Design review of the part built by this model. Coordinates are the model's own, in mm. Face numbers are marked on the shaded views. A direction names the side the tool comes from. Coordinates: 2 decimals unless noted, no trailing zeros. Loops run counter-clockwise (first coordinate to the right, second up) from the corner with the lowest first, then second, coordinate; pieces in that order, holes last. Notation, with made-up numbers: (46, -38.5) -> (75, -38.5) arc R5 ccw to (75, -34.5) -> close; hole circle Ø2 at (80, 70). An arc over 180 degrees is marked (long way). One line per item, written item: value. Start each with the question number.
1. Add section B-B on y = 15. Write out the cut boundary in (x, z).
2. Add section C-C on z = 3. Write out the cut boundary in (x, y), plus the area to 3 significant figures.
3. Add section A-A on z = -2.5. Write out the cut boundary in (x, y), plus the area to 3 significant figures.
4. Machinability: for the marked faces 1 and 2, which of the approach directions +Z, -Z, +X, -X, +Y, -Y give a long, thin tool a straight path to every point of the face, cutting with its end or side? Answer none if there is none.
5. Insertion check: pin 1 (2.5 mm diameter, centred on y = 11.14, z = 21.82, fed in from -X); pin 2 (1 mm diameter, centred on x = -1.5, y = -0.5, fed in from +Z); pin 3 (2 mm diameter, centred on y = 15, z = 25, fed in from -X); pin 4 (1.5 mm diameter, centred on x = -0.5, z = 19, fed in from +Y). Each pin has a flat end and moves straight along its axis. Give the tip position at first contact, or say it passes through.
6. For probe 1 along Z at (x, y) = (-0.35, 16); probe 2 along Z at (x, y) = (-1.25, 14); probe 3 along Y at (x, z) = (0.65, 18.5), list the stretches that pass through material, from the lowest coordinate up.
7. Add section D-D on x = -1.9. Write out the cut boundary in (y, z) (3 decimals).
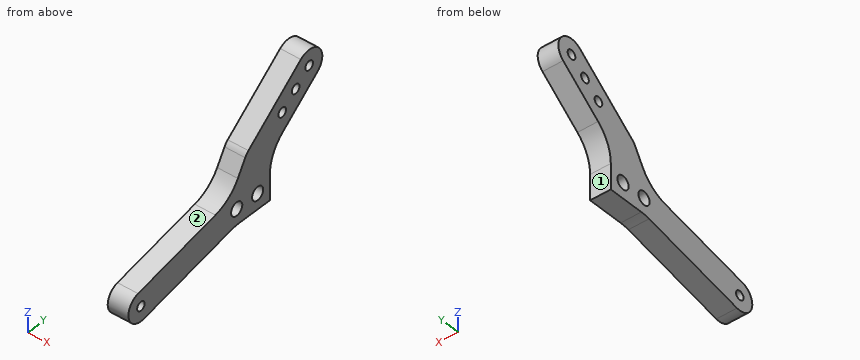
```python
from build123d import *

# Parameters (mm, degrees)
SKETCH1_W           = 5
SKETCH1_H           = 7.5
BOSS_EXTRUDE1_DEPTH = 13
BOSS_EXTRUDE4_DEPTH = 5
SKETCH2_R           = 1.1
CUT_EXTRUDE1_DEPTH  = 35.686092314
LPATTERN1_COUNT     = 3
LPATTERN1_PITCH     = 5
SKETCH3_R           = 1.6
CUT_EXTRUDE2_DEPTH  = 35.686092314
BOSS_EXTRUDE2_DEPTH = 5
LPATTERN2_COUNT     = 2
LPATTERN2_PITCH     = 6
SKETCH5_R           = 1.075
SKETCH5_R_2         = 1.6
BOSS_EXTRUDE3_DEPTH = 5
FILLET2_R           = 10


with BuildPart() as part:
    # Sketch1 → Boss-Extrude1 (new body)
    with BuildSketch(Plane.XY):
        Rectangle(SKETCH1_W, SKETCH1_H)
    extrude(amount=BOSS_EXTRUDE1_DEPTH)

    # Sketch6 → Boss-Extrude4 (add)
    with BuildSketch(Plane(origin=(2.5, 0, 0), x_dir=(0, 0, -1), z_dir=(1, 0, 0))):
        with BuildLine():
            Line((-15.501719728, -2.388104729), (-27.89127235, 12.611895271))
            ThreePointArc((-27.89127235, 12.611895271), (-27.388104729, 17.89127235), (-22.10872765, 17.388104729))
            Line((-22.10872765, 17.388104729), (-9.719175027, 2.388104729))
            ThreePointArc((-9.719175027, 2.388104729), (-10.222342649, -2.89127235), (-15.501719728, -2.388104729))
        make_face()
    extrude(amount=-BOSS_EXTRUDE4_DEPTH)

    # Sketch2 → Cut-Extrude1 (cut, through all)
    with BuildSketch(Plane(origin=(2.5, 0, 0), x_dir=(0, 0, -1), z_dir=(1, 0, 0))):
        with Locations((-25, 15)):
            Circle(SKETCH2_R)
    cut_extrude1 = extrude(amount=-CUT_EXTRUDE1_DEPTH, mode=Mode.SUBTRACT)

    # LPattern1: Cut-Extrude1 ×3
    with Locations(*[Vector(0, -0.7710059601120912, -0.6368279276787667) * (i * LPATTERN1_PITCH) for i in range(1, LPATTERN1_COUNT)]):
        add(cut_extrude1, mode=Mode.SUBTRACT)

    # Sketch3 → Cut-Extrude2 (cut, through all)
    with BuildSketch(Plane(origin=(2.5, 0, 0), x_dir=(0, 0, -1), z_dir=(1, 0, 0))):
        with Locations((-3.75, 0.25)):
            Circle(SKETCH3_R)
    cut_extrude2 = extrude(amount=-CUT_EXTRUDE2_DEPTH, mode=Mode.SUBTRACT)

    # Sketch4 → Boss-Extrude2 (add)
    with BuildSketch(Plane(origin=(2.5, 0, 0), x_dir=(0, 0, -1), z_dir=(1, 0, 0))):
        Polygon((0, -3.75), (0, -8.75), (-5, -8.75), (-14.382714397, -3.304779813), align=None)
    extrude(amount=-BOSS_EXTRUDE2_DEPTH)

    # LPattern2: Cut-Extrude2 ×2
    with Locations(*[(0, -i * LPATTERN2_PITCH, 0) for i in range(1, LPATTERN2_COUNT)]):
        add(cut_extrude2, mode=Mode.SUBTRACT)

    # Sketch5 → Boss-Extrude3 (add)
    with BuildSketch(Plane(origin=(2.5, 0, 0), x_dir=(0, 0, -1), z_dir=(1, 0, 0))):
        with BuildLine():
            Line((-0.985537893, -33.954911928), (-7.235537893, -6.544764489))
            ThreePointArc((-7.235537893, -6.544764489), (-4.544764489, -2.264462107), (-0.264462107, -4.955235511))
            Line((-0.264462107, -4.955235511), (5.985537893, -32.365382949))
            ThreePointArc((5.985537893, -32.365382949), (3.294764489, -36.645685332), (-0.985537893, -33.954911928))
        make_face()
        with Locations((2.5, -33.160147439)):
            Circle(SKETCH5_R, mode=Mode.SUBTRACT)
        with Locations((-3.75, -5.75)):
            Circle(SKETCH5_R_2, mode=Mode.SUBTRACT)
    extrude(amount=-BOSS_EXTRUDE3_DEPTH)

    # Fillet2
    fillet2_edges = [part.edges().sort_by_distance(p)[0] for p in [
        (0, 3.75, 10.844059902),
        (0, -7.591071621, 6.996961301),
        (0, -6.115066764, 0),
    ]]
    fillet(fillet2_edges, radius=FILLET2_R)


solid = part.part
```
Worked answers:
1. outline: (-2.5, 20.14) -> (2.5, 20.14) -> (2.5, 23.9) -> (-2.5, 23.9) -> close; (-2.5, 26.1) -> (2.5, 26.1) -> (2.5, 28.75) -> (-2.5, 28.75) -> close
2. outline: (-2.5, -25.12) -> (2.5, -25.12) -> (2.5, -7.16) -> (-2.5, -7.16) -> close; (-2.5, -4.34) -> (2.5, -4.34) -> (2.5, -1.16) -> (-2.5, -1.16) -> close; (-2.5, 1.66) -> (2.5, 1.66) -> (2.5, 3.75) -> (-2.5, 3.75) -> close
2. area: 116 mm²
3. outline: (-2.5, -36.74) -> (2.5, -36.74) -> (2.5, -34.24) -> (-2.5, -34.24) -> close; (-2.5, -32.09) -> (2.5, -32.09) -> (2.5, -17.08) -> (-2.5, -17.08) -> close
3. area: 87.5 mm²
4. face 1: -Z, +X, -X, +Y
4. face 2: +Z, +X, -X, -Y
5. pin 1: stops at x = -2.5
5. pin 2: stops at z = 17.47
5. pin 3: passes through
5. pin 4: stops at y = 14.53
6. probe 1: z = 20.96 to 24.54, 25.46 to 28.61
6. probe 2: z = 19.31 to 24.54, 25.46 to 28.61
6. probe 3: y = 1.24 to 6.2, 8.38 to 13.02
7. outline: (-33.955, 0.986) arc R3.575 ccw to (-32.365, -5.986) -> (-7.213, -0.25) arc R10 cw to (-4.989, 0) -> (3.75, 0) -> (3.75, 6.134) arc R10 cw to (7.382, 13.844) -> (17.388, 22.109) arc R3.75 ccw to (12.612, 27.891) -> (-2.388, 15.502) arc R3.75 ccw to (-3.305, 14.383) -> (-5.407, 10.76) arc R10 cw to (-11.833, 6.03) -> close; hole circle Ø2.15 at (-33.16, -2.5); hole circle Ø3.2 at (-5.75, 3.75); hole circle Ø3.2 at (0.25, 3.75); hole circle Ø2.2 at (7.29, 18.632); hole circle Ø2.2 at (11.145, 21.816); hole circle Ø2.2 at (15, 25)
